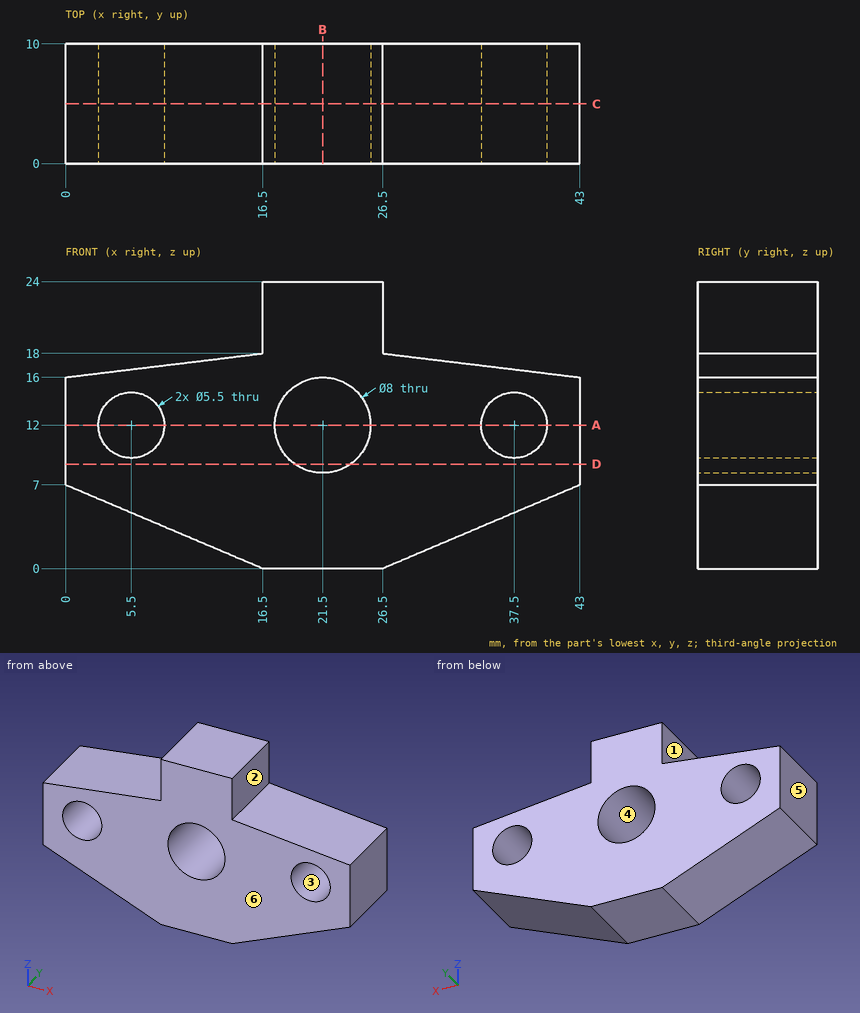
Check sheet for the drawn part. Datum: minimum x, y, z corner. Units: mm. A direction names the side the tool comes from. Give positions to 0.01 mm unless a question says otherwise; leave off trailing zeros. Order: outer loops, then holes, each group sorted by start corner. A loop starts at its lowest first (then second) coordinate and runs counter-clockwise, first axis right, second up. Notation, with made-up numbers: (63.5, 52.5) - (121.5, 52.5) arc R21 ccw to (121.5, 79.5) - close; hole circle Ø11 at (6.5, 51.25). An arc over 180 degrees is marked (long way). Answer as a JSON object with one key per item and string values.
(1) Material ranges on line 1 (X direction, y = 3.25, z = 12); line 2 (X direction, y = 5.5, z = 14.5); line 3 (Z direction, x = 36, y = 1.5), recorded low to high.
Report:
{"line 1": "0 to 2.75, 8.25 to 17.5, 25.5 to 34.75, 40.25 to 43", "line 2": "0 to 4.35, 6.65 to 18.38, 24.62 to 36.35, 38.65 to 43", "line 3": "4.03 to 9.7, 14.3 to 16.85"}
(2) Tool access check on the marked faces 1, 2 and 3. Record the directions out of +Z, -Z, +X, -X, +Y, -Y that give a thin tool (end or side, any length) a straight path to the whole face; none if there is none.
Report:
{"face 1": "+Z, -X, +Y, -Y", "face 2": "+Z, +X, +Y, -Y", "face 3": "+Y, -Y"}
(3) Cross-section at D-D (z = 8.75). Record the cut outline in (x, y), then the cut area to 3 significant figures.
Report:
{"outline": "(0, 0) - (19.17, 0) - (19.17, 10) - (0, 10) - close; (23.83, 0) - (43, 0) - (43, 10) - (23.83, 10) - close", "area": "383 mm^2"}
(4) Cross-section at B-B (x = 21.5). Record the cut outline in (y, z), then the cut area to 3 significant figures.
Report:
{"outline": "(0, 0) - (10, 0) - (10, 8) - (0, 8) - close; (0, 16) - (10, 16) - (10, 24) - (0, 24) - close", "area": "160 mm^2"}
(5) Cross-section at C-C (y = 5). Record the cut outline in (x, z).
Report:
{"outline": "(0, 7) - (16.5, 0) - (26.5, 0) - (43, 7) - (43, 16) - (26.5, 18) - (26.5, 24) - (16.5, 24) - (16.5, 18) - (0, 16) - close; hole circle Ø5.5 at (5.5, 12); hole circle Ø8 at (21.5, 12); hole circle Ø5.5 at (37.5, 12)"}
(6) Draft check along X on the marked faces 4, 5 and 6. Enter one of: released by +X, released by -X, zero draft, split by the parting line, or undercut.
Report:
{"face 4": "undercut", "face 5": "released by -X", "face 6": "zero draft"}
(7) Depth check by flat-ended pin: pin 1 Ø3 at (x, y) = (38.5, 4) entering from +Z; pin 2 Ø5 at (y, z) = (3.5, 21) entering from -X; pin 3 Ø1 at (y, z) = (8.5, 4) entering from +X. Enter the tip coordinate at first touch or a pass-through.
Report:
{"pin 1": "z = 16.73", "pin 2": "x = 16.5", "pin 3": "x = 37.11"}
(8) Cross-section at A-A (z = 12). Record the cut outline in (x, y).
Report:
{"outline": "(0, 0) - (2.75, 0) - (2.75, 10) - (0, 10) - close; (8.25, 0) - (17.5, 0) - (17.5, 10) - (8.25, 10) - close; (25.5, 0) - (34.75, 0) - (34.75, 10) - (25.5, 10) - close; (40.25, 0) - (43, 0) - (43, 10) - (40.25, 10) - close"}
